Could you check a few things on this model? Use its own coordinates, in mm. Face numbers are marked on the shaded views. A direction names the side the tool comes from. Coordinates: 2 decimals unless noted, no trailing zeros. Write each loop counter-clockwise with the first axis right and the second up, starting at its lowest first coordinate (ties: lowest second). Pieces come first, ordered by that corner, then holes. Notation, with made-up numbers: (-17.75, -7) - (8.25, -7) arc R33 cw to (8.25, 30) - close; hole circle Ø1 at (29.5, 16). An arc over 180 degrees is marked (long way). Answer as a JSON object with one key per item and string values. Group by question number.
1) Please list where these lines run through material, in increasing order: line 1 along Y through (x, z) = (639, 284.5); line 2 along X through (y, z) = (165, 233.5); line 3 along X through (y, z) = (340, 38).
2) If we section it at A-A (y = 427): Write out the boundary of the cut face in (x, z), plus the area to 3 significant figures.
3) We'd pull the mould along Y, two halves only. Please class the marked faces 1, 2, 3 and 4: released by +Y, released by -Y, zero draft, split by the parting line, or undercut.
4) Will this pin go through, and if not, where does the flat tip stop? pin 1 Ø4 at (x, y) = (90, 280.5) entering from +Z.
5) If we section it at B-B (x = 652): Write out the boundary of the cut face in (y, z).
6) On a 3-axis mill with a long thin cutter (end or side, diameter ignored), from which of +Z, -Z, +X, -X, +Y, -Y can I reach the whole of each face in a straight line? I mean the marked faces 5 and 6. Say none if no direction works.
7) If we section it at C-C (z = 239): State how many separate pieces and enclosed holes the cut face has, plus the area to 3 significant figures.
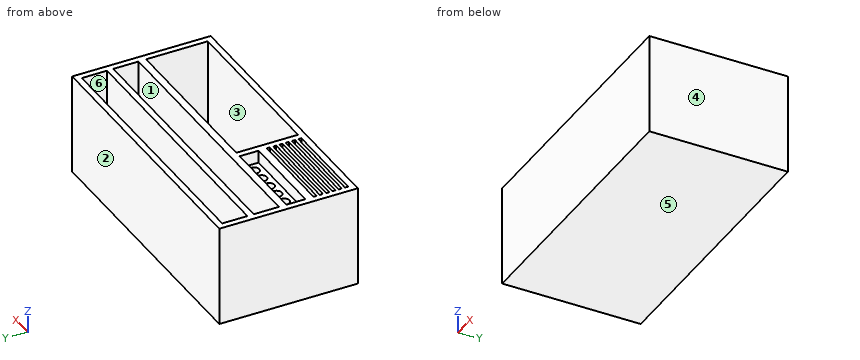
```python
from build123d import *

# Parameters (mm, degrees)
F0_W     = 1117.6
F0_H     = 558.8
F1_DEPTH = 406.4
F2_W     = 355.6
F2_H     = 12.7
F2_W_2   = 1066.8
F2_H_2   = 101.6
F2_W_3   = 685.8
F2_H_3   = 248.804872
F3_DEPTH = 381
F4_W     = 355.6
F4_H     = 76.2
F5_DEPTH = 50.8
F6_R     = 20.6375
F7_DEPTH = 101.6


with BuildPart() as f1:
    # F0 (on Top) → F1 (new body)
    with BuildSketch(Plane.XY):
        with Locations((466.017957, 231.267335)):
            Rectangle(F0_W, F0_H)
    extrude(amount=F1_DEPTH)

    # F2 (on face) → F3 (cut)
    with BuildSketch(Plane.XY.offset(406.4)):
        with Locations((110.417957, -16.382665)):
            Rectangle(F2_W, F2_H)
        with Locations((110.417957, 9.017335)):
            Rectangle(F2_W, F2_H)
        with Locations((110.417957, 34.417335)):
            Rectangle(F2_W, F2_H)
        with Locations((110.417957, 59.817335)):
            Rectangle(F2_W, F2_H)
        with Locations((110.417957, 85.217335)):
            Rectangle(F2_W, F2_H)
        with Locations((110.417957, 110.617335)):
            Rectangle(F2_W, F2_H)
        with Locations((466.017957, 434.467335)):
            Rectangle(F2_W_2, F2_H_2)
        with Locations((466.017957, 307.467335)):
            Rectangle(F2_W_2, F2_H_2)
        with Locations((656.517957, 101.669771)):
            Rectangle(F2_W_3, F2_H_3)
    extrude(amount=-F3_DEPTH, mode=Mode.SUBTRACT)

    # F4 (on face) → F5 (cut)
    with BuildSketch(Plane.XY.offset(406.4)):
        with Locations((110.417957, 187.972207)):
            Rectangle(F4_W, F4_H)
    extrude(amount=-F5_DEPTH, mode=Mode.SUBTRACT)

    # F6 (on face) → F7 (cut)
    with BuildSketch(Plane.XY.offset(355.6)):
        with Locations((-35.632043, 187.972207)):
            Circle(F6_R)
        with Locations((21.517957, 187.972207)):
            Circle(F6_R)
        with Locations((78.667957, 187.972207)):
            Circle(F6_R)
        with Locations((135.817957, 187.972207)):
            Circle(F6_R)
        with Locations((192.967957, 187.972207)):
            Circle(F6_R)
        with Locations((250.117957, 187.972207)):
            Circle(F6_R)
    extrude(amount=-F7_DEPTH, mode=Mode.SUBTRACT)


solid = f1.part
```
Here are the results:
{
 "1": {"line 1": "y = -48.13 to -22.73, 226.07 to 256.67, 358.27 to 383.67, 485.27 to 510.67", "line 2": "x = -92.78 to 313.62, 999.42 to 1024.82", "line 3": "x = -92.78 to -67.38, 999.42 to 1024.82"},
 "2": {"outline": "(-92.78, 0) - (1024.82, 0) - (1024.82, 406.4) - (999.42, 406.4) - (999.42, 25.4) - (-67.38, 25.4) - (-67.38, 406.4) - (-92.78, 406.4) - close", "area": "47,700 mm²"},
 "3": {"face 1": "undercut", "face 2": "released by +Y", "face 3": "undercut", "face 4": "zero draft"},
 "4": {"pin 1": "stops at z = 25.4"},
 "5": {"outline": "(-48.13, 0) - (510.67, 0) - (510.67, 406.4) - (485.27, 406.4) - (485.27, 25.4) - (383.67, 25.4) - (383.67, 406.4) - (358.27, 406.4) - (358.27, 25.4) - (256.67, 25.4) - (256.67, 406.4) - (226.07, 406.4) - (226.07, 25.4) - (-22.73, 25.4) - (-22.73, 406.4) - (-48.13, 406.4) - close"},
 "6": {"face 5": "-Z, +X, -X, +Y, -Y", "face 6": "+Z"},
 "7": {"separate pieces": "1", "enclosed holes": "9", "area": "210,000 mm²"}
}
